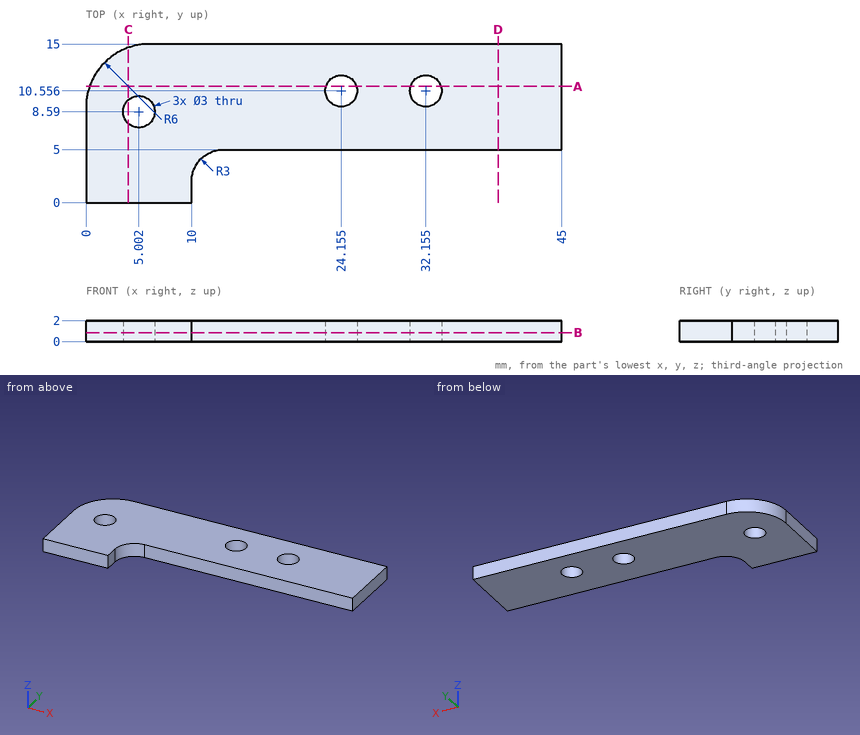
Input: dimensioned drawing with shaded views. Units: mm. Origin: part minimum x, y, z. Coordinates: 2 decimals unless noted, no trailing zeros. Write each loop counter-clockwise with the first axis right and the second up, starting at its lowest first coordinate (ties: lowest second). Pieces come first, ordered by that corner, then holes. Notation, with made-up numbers: M 81.5,31 L 136.5,31 A35 ccw 136.5,70 Z; hole C 26.25,-37.5 d11. An arc over 180 degrees is marked long. Use a Markdown table: item, result.
1) Section A-A, the plane y = 11. Output: boundary loops of the cut face in (x, z).
Conclusion:
| item | result |
|---|---|
| outline | M 0.34,0 L 22.72,0 L 22.72,2 L 0.34,2 Z; M 25.59,0 L 30.72,0 L 30.72,2 L 25.59,2 Z; M 33.59,0 L 45,0 L 45,2 L 33.59,2 Z |
2) Ray query, L1, parallel to Y at x = 16, z = 0.7; L2, parallel to Y at x = 5, z = 1 (1 decimal); L3, parallel to Y at x = 25.5, z = 1.4 (1 decimal). Return the intervals inside material, ascending.
Conclusion:
| item | result |
|---|---|
| L1 | y = 5 to 15 |
| L2 | y = 0 to 7.1, 10.1 to 14.9 |
| L3 | y = 5 to 9.9, 11.2 to 15 |
3) Section D-D, the plane x = 39. Output: boundary loops of the cut face in (y, z), then the cut area to 3 significant figures.
Conclusion:
| item | result |
|---|---|
| outline | M 5,0 L 15,0 L 15,2 L 5,2 Z |
| area | 20.0 mm^2 |
4) Section B-B, the plane z = 0.85. Output: boundary loops of the cut face in (x, y) (1 decimal).
Conclusion:
| item | result |
|---|---|
| outline | M 0,0 L 10,0 L 10,2 A3 cw 13,5 L 45,5 L 45,15 L 6,15 A6 ccw 0,9 Z; hole C 5,8.6 d3; hole C 24.2,10.6 d3; hole C 32.2,10.6 d3 |
5) Section C-C, the plane x = 4. Output: boundary loops of the cut face in (y, z).
Conclusion:
| item | result |
|---|---|
| outline | M 0,0 L 7.47,0 L 7.47,2 L 0,2 Z; M 9.71,0 L 14.66,0 L 14.66,2 L 9.71,2 Z |
6) First-contact query: pin 1 Ø5 at (x, y) = (24.16, 10.56) entering from -Z. Flat tip, straight axial feed; report the tip coordinate or a pass-through.
Conclusion:
| item | result |
|---|---|
| pin 1 | stops at z = 0 |
